```python
from build123d import *

# Parameters (mm, degrees)
CROQUIS1_W              = 23.5
CROQUIS1_H              = 5
CROQUIS1_W_2            = 20.5
CROQUIS1_H_2            = 2
SALIENTE_EXTRUIR1_DEPTH = 20
CROQUIS5_W              = 15
CROQUIS5_H              = 18.5
SALIENTE_EXTRUIR3_DEPTH = 10.2
CROQUIS6_W              = 15.8
CROQUIS6_H              = 8.2
CORTAR_EXTRUIR2_DEPTH   = 15
REDONDEO3_R             = 1.5
CORTAR_EXTRUIR3_DEPTH   = 3
REDONDEO4_R             = 1
REDONDEO5_R             = 1.5


with BuildPart() as part:
    # Croquis1 → Saliente-Extruir1 (new body)
    with BuildSketch(Plane.XY):
        with Locations((-10.25, 1)):
            Rectangle(CROQUIS1_W, CROQUIS1_H)
        with Locations((-10.25, 1)):
            Rectangle(CROQUIS1_W_2, CROQUIS1_H_2, mode=Mode.SUBTRACT)
    extrude(amount=SALIENTE_EXTRUIR1_DEPTH)

    # Croquis5 → Saliente-Extruir3 (add)
    with BuildSketch(Plane.XZ.offset(1.5)):
        with Locations((-10.25, 10)):
            Rectangle(CROQUIS5_W, CROQUIS5_H)
    extrude(amount=SALIENTE_EXTRUIR3_DEPTH)

    # Croquis6 → Cortar-Extruir2 (cut)
    with BuildSketch(Plane.ZY.offset(17.75)):
        with Locations((10, -6.4)):
            Rectangle(CROQUIS6_W, CROQUIS6_H)
    extrude(amount=-CORTAR_EXTRUIR2_DEPTH, mode=Mode.SUBTRACT)

    # Redondeo3
    redondeo3_edges = [part.edges().sort_by_distance(p)[0] for p in [
        (-10.25, -2.3, 17.9),
        (-10.25, -10.5, 17.9),
    ]]
    fillet(redondeo3_edges, radius=REDONDEO3_R)

    # Croquis7 → Cortar-Extruir3 (cut)
    with BuildSketch(Plane.ZY.offset(17.75)):
        with BuildLine():
            Line((17.9, -11), (2.1, -11))
            ThreePointArc((2.1, -11), (1.746446609, -10.853553391), (1.6, -10.5))
            Line((1.6, -10.5), (1.6, -2.3))
            ThreePointArc((1.6, -2.3), (1.746446609, -1.946446609), (2.1, -1.8))
            Line((2.1, -1.8), (17.9, -1.8))
            ThreePointArc((17.9, -1.8), (18.253553391, -1.946446609), (18.4, -2.3))
            Line((18.4, -2.3), (18.4, -10.5))
            ThreePointArc((18.4, -10.5), (18.253553391, -10.853553391), (17.9, -11))
        make_face()
    extrude(amount=-CORTAR_EXTRUIR3_DEPTH, mode=Mode.SUBTRACT)

    # Redondeo4
    # the kernel refuses this fillet: 1 mm, written as the material it adds along each edge
    with BuildSketch(Plane(origin=(-2.75, -1.5, 0.75), x_dir=(0, 0, -1), z_dir=(-1, 0, 0))) as redondeo4_piece_1:
        with BuildLine():
            CenterArc((1, 0.968245837), REDONDEO4_R, 180, 75.522487814)
            Line((0, 0.968245837), (0, 0))
            Line((0, 0), (0.75, 0))
        make_face()
    extrude(amount=15)
    with BuildSketch(Plane(origin=(-17.75, -1.5, 19.25), x_dir=(0, -1, 0), z_dir=(1, 0, 0))) as redondeo4_piece_2:
        with BuildLine():
            CenterArc((0.968245837, -1), REDONDEO4_R, 90, 75.522487814)
            Line((0, -0.75), (0, 0))
            Line((0, 0), (0.968245837, 0))
        make_face()
    extrude(amount=15)
    # the kernel refuses this fillet: 1 mm, written as the material it takes off along each edge
    with BuildSketch(Plane(origin=(-0.25, -11.7, 0.75), x_dir=(0, 1, 0), z_dir=(-1, 0, 0))) as redondeo4_2_piece_1:
        with BuildLine():
            CenterArc((REDONDEO4_R, -REDONDEO4_R), REDONDEO4_R, 90, 90)
            Line((0, -REDONDEO4_R), (0, 0))
            Line((0, 0), (REDONDEO4_R, 0))
        make_face()
    extrude(amount=20, mode=Mode.SUBTRACT)
    with BuildSketch(Plane(origin=(-20.25, -11.7, 19.25), x_dir=(0, 0, -1), z_dir=(1, 0, 0))) as redondeo4_2_piece_2:
        with BuildLine():
            CenterArc((REDONDEO4_R, REDONDEO4_R), REDONDEO4_R, 180, 90)
            Line((0, REDONDEO4_R), (0, 0))
            Line((0, 0), (REDONDEO4_R, 0))
        make_face()
    extrude(amount=20, mode=Mode.SUBTRACT)

    # Redondeo5
    redondeo5_edges = [part.edges().sort_by_distance(p)[0] for p in [
        (-22, -1.5, 10),
        (-22, 3.5, 10),
        (1.5, 3.5, 10),
        (1.5, -1.5, 10),
    ]]
    fillet(redondeo5_edges, radius=REDONDEO5_R)


solid = part.part
```
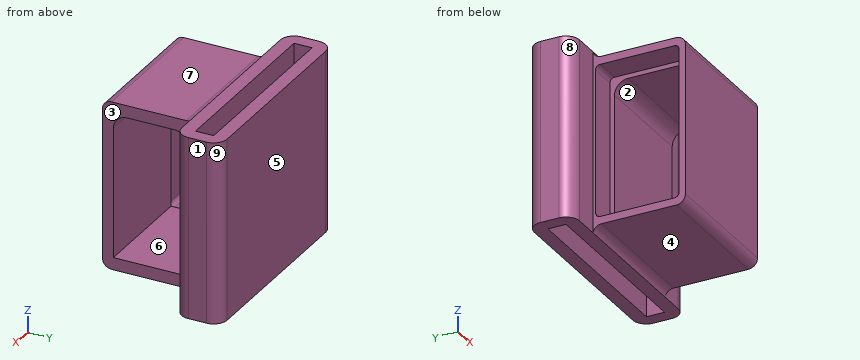
Could you check a few things on this model? Use its own coordinates, in mm. Face numbers are marked on the shaded views. A direction names the side the tool comes from. Give positions to 0.01 mm unless a question says otherwise; leave off trailing zeros. Order: outer loops, then holes, each group sorted by start corner. A loop starts at its lowest first (then second) coordinate and runs counter-clockwise, first axis right, second up.
Q1. I'm going to push flat-ended pins straight in: P1, Ø0.8, axis at x = -0.5, z = 7.5, coming from the -Y side; P2, Ø8, axis at x = -6, y = -4, coming from the -Z side; P3, Ø4.5, axis at y = -6.5, z = 7, coming from the -X side; P4, Ø2, axis at y = -7.5, z = 17, coming from the -X side. Where does each tip first touch, or does it pass through?
Q2. Suppose I cut it at D-D, the plane y = -6.25. Write out the boundary of the cut face in (x, z), and give its area (3 significant figures).
Q3. If I drill on line 1 along Y through (x, z) = (-10.25, 14.75); line 2 along Y through (x, z) = (-2.5, 8.75); line 3 along Z through (x, y) = (-17, -7.5), over which ranges is the centre line in solid material (lowest first)?
Q4. Suppose I cut it at A-A, the plane x = -6.75. Write out the boundary of the cut face in (y, z), and give its area (3 significant figures).
Q5. We'd pull the mould along Y, two halves only. Please class the marked faces 6, 7, 8 and 9: +Y half, -Y half, draft (parallel to the pull), parting line (faces both ways), or undercut.
Q6. For the marked faces 1, 2, 3, 4 and 5, which set-ups out of +Z, -Z, +X, -X, +Y, -Y let a thin tool reach every point of the face, with its end or its side?
Q7. Suppose I cut it at C-C, the plane x = -19. Write out the boundary of the cut face in (y, z).
Q8. Suppose I cut it at B-B, the plane z = 8.25. Write out the boundary of the cut face in (x, y).
Solution:
1. P1: stops at y = -1.5
1. P2: stops at z = 0
1. P3: passes through
1. P4: stops at x = -14.75
2. outline: (-17.75, 0.75) - (-2.75, 0.75) - (-2.75, 2.1) - (-14.75, 2.1) - (-14.75, 1.6) - (-17.75, 1.6) - close; (-17.75, 18.4) - (-14.75, 18.4) - (-14.75, 17.9) - (-2.75, 17.9) - (-2.75, 19.25) - (-17.75, 19.25) - close
2. area: 37.5 mm2
3. line 1: y = -11.7 to -10.5, -2.3 to 0, 2 to 3.5
3. line 2: y = -1.5 to 0, 2 to 3.5
3. line 3: z = 0.75 to 1.6, 18.4 to 19.25
4. outline: (-11.7, 1.75) arc R1 ccw to (-10.7, 0.75) - (-2.47, 0.75) arc R1 cw to (-1.5, 0) - (0, 0) - (0, 20) - (-1.5, 20) arc R1 cw to (-2.47, 19.25) - (-10.7, 19.25) arc R1 ccw to (-11.7, 18.25) - close; (2, 0) - (3.5, 0) - (3.5, 20) - (2, 20) - close; hole (-10.5, 2.1) - (-2.3, 2.1) - (-2.3, 16.4) arc R1.5 ccw to (-3.8, 17.9) - (-9, 17.9) arc R1.5 ccw to (-10.5, 16.4) - close
4. area: 120 mm2
5. face 6: undercut
5. face 7: draft
5. face 8: -Y half
5. face 9: +Y half
6. face 1: +Z, -Z, +X, +Y, -Y
6. face 2: +X, -X
6. face 3: +Z, -Z, +X, -Y
6. face 4: -Z, +X, -X, -Y
6. face 5: +Z, -Z, +X, -X, +Y
7. outline: (-1.5, 0) - (0, 0) - (0, 20) - (-1.5, 20) - close; (2, 0) - (3.5, 0) - (3.5, 20) - (2, 20) - close
8. outline: (-22, 0) arc R1.5 ccw to (-20.5, -1.5) - (-17.75, -1.5) - (-17.75, -1.8) - (-14.75, -1.8) - (-14.75, -2.3) - (-2.75, -2.3) - (-2.75, -1.5) - (0, -1.5) arc R1.5 ccw to (1.5, 0) - (1.5, 2) arc R1.5 ccw to (0, 3.5) - (-20.5, 3.5) arc R1.5 ccw to (-22, 2) - close; (-17.75, -11.7) - (-2.75, -11.7) - (-2.75, -10.5) - (-14.75, -10.5) - (-14.75, -11) - (-17.75, -11) - close; hole (-20.5, 0) - (0, 0) - (0, 2) - (-20.5, 2) - close
